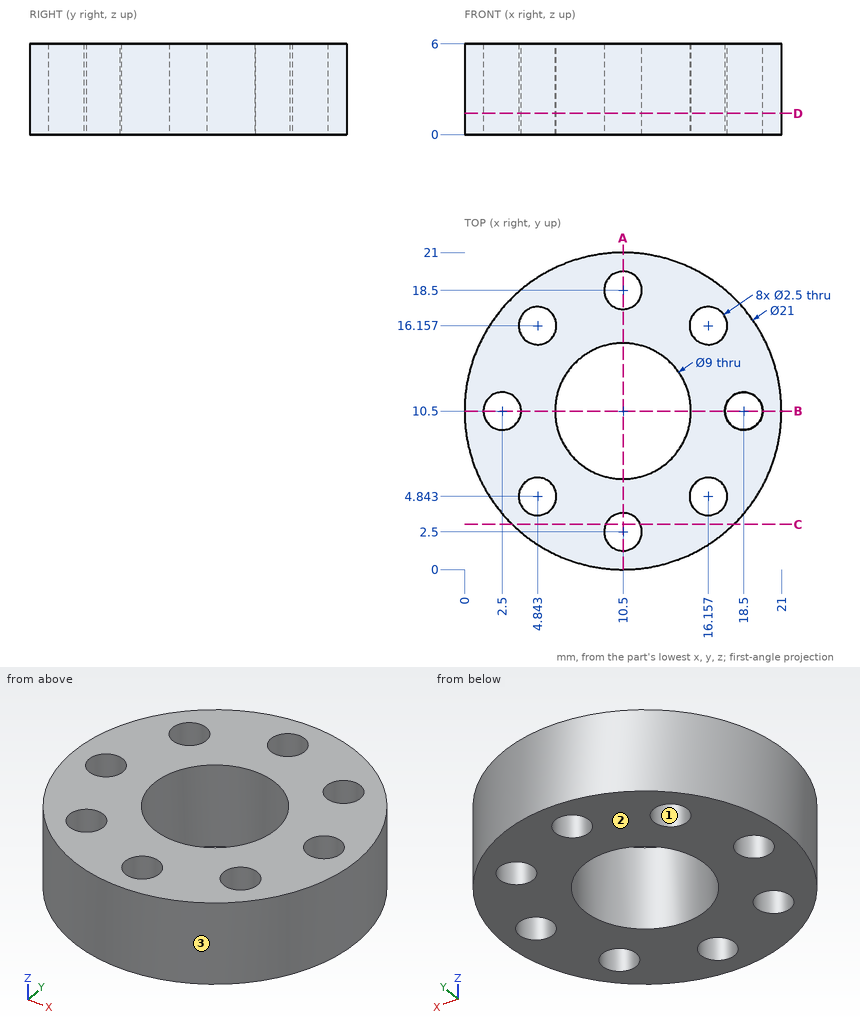
Source: three-view drawing plus pictorial views. Frame: mm from the lowest corner of the part. Coordinates: 2 decimals unless noted, no trailing zeros. Loops run counter-clockwise (first coordinate to the right, second up) from the corner with the lowest first, then second, coordinate; pieces in that order, holes last. Notation, with made-up numbers: (-29.75, 45.5) - (-24.75, 45.5) arc R25 cw to (-24.75, 83.5) - close; hole circle Ø4 at (59, 81.5). An arc over 180 degrees is marked (long way). Answer in a Markdown table with one row per item. Add a question column.
Item 1: Contact query for a flat-ended pin moving along its axis: P1, Ø3, axis at x = 6, z = 1.5, coming from the +Y side. Output: stop coordinate, or through.
Item 2: Section query A-A on x = 10.5. Return the cut outline in (y, z), then the cut area to 3 significant figures.
Item 3: Mould query, pull axis Y, two halves, no side actions, for the marked faces 1, 2 and 3. Classes: released by +Y, released by -Y, zero draft, split by the parting line, or undercut.
Item 4: Section query C-C on y = 3. Return the cut outline in (x, z).
Item 5: Line query: line 1 along Y through (x, z) = (5.75, 2.95); line 2 along Y through (x, z) = (4.5, 1.8) (1 decimal); line 3 along X through (y, z) = (8.25, 3.2). Output: solid intervals per line, ascending. Write a range as [from, to].
Item 6: Section query D-D on z = 1.4. State how many separate pieces and enclosed holes the cut face has.
Recorded:
| question | item | result |
|---|---|---|
| 1 | P1 | y = 20.56 |
| 2 | outline | (0, 0) - (1.25, 0) - (1.25, 6) - (0, 6) - close; (3.75, 0) - (6, 0) - (6, 6) - (3.75, 6) - close; (15, 0) - (17.25, 0) - (17.25, 6) - (15, 6) - close; (19.75, 0) - (21, 0) - (21, 6) - (19.75, 6) - close |
| 2 | area | 42.0 mm^2 |
| 3 | face 1 | undercut |
| 3 | face 2 | zero draft |
| 3 | face 3 | split by the parting line |
| 4 | outline | (3.15, 0) - (9.35, 0) - (9.35, 6) - (3.15, 6) - close; (11.65, 0) - (17.85, 0) - (17.85, 6) - (11.65, 6) - close |
| 5 | line 1 | [1.14, 3.98], [5.7, 15.3], [17.02, 19.86] |
| 5 | line 2 | [1.9, 3.6], [6, 15], [17.4, 19.1] |
| 5 | line 3 | [0.24, 6.6], [14.4, 20.76] |
| 6 | separate pieces | 1 |
| 6 | enclosed holes | 9 |
